Design review of the part built by this model. Coordinates are the model's own, in mm. A direction names the side the tool comes from. Give positions to 0.01 mm unless a question says otherwise; leave off trailing zeros. Loops run counter-clockwise (first coordinate to the right, second up) from the corner with the lowest first, then second, coordinate; pieces in that order, holes last. Notation, with made-up numbers: M 70.25,-33 L 111.25,-33 A19 cw 111.25,-17 Z; hole C 49.5,69.5 d11. An arc over 180 degrees is marked long. Answer as CSV lines item,"result".
```python
from build123d import *

# Parameters (mm, degrees)
SKETCH1_R           = 11
SKETCH1_R_2         = 4
BOSS_EXTRUDE1_DEPTH = 3.5
SKETCH2_R           = 9.4
SKETCH2_R_2         = 5.875
CUT_EXTRUDE1_DEPTH  = 0.5
CUT_EXTRUDE2_START  = -1
SKETCH3_R           = 9.4
SKETCH3_R_2         = 5.875
CUT_EXTRUDE2_DEPTH  = 1
CHAMFER1_SIZE       = 0.5


with BuildPart() as part:
    # Sketch1 → Boss-Extrude1 (new, symmetric)
    with BuildSketch(Plane.XY):
        Circle(SKETCH1_R)
        Circle(SKETCH1_R_2, mode=Mode.SUBTRACT)
    extrude(amount=BOSS_EXTRUDE1_DEPTH, both=True)

    # Sketch2 → Cut-Extrude1 (cut)
    with BuildSketch(Plane.XY.offset(3.5)):
        Circle(SKETCH2_R)
        Circle(SKETCH2_R_2, mode=Mode.SUBTRACT)
    extrude(amount=-CUT_EXTRUDE1_DEPTH, mode=Mode.SUBTRACT)

    # Sketch3 → Cut-Extrude2 (cut)
    with BuildSketch(Plane(origin=(0, 0, -3.5), x_dir=(-1, 0, 0), z_dir=(0, 0, -1)).offset(CUT_EXTRUDE2_START)):
        with Locations(Location((0, 0, 0), (0, 0, 180))):
            Circle(SKETCH3_R)
        with Locations(Location((0, 0, 0), (0, 0, 180))):
            Circle(SKETCH3_R_2, mode=Mode.SUBTRACT)
    extrude(amount=CUT_EXTRUDE2_DEPTH, mode=Mode.SUBTRACT)

    # Chamfer1
    chamfer1_edges = [part.edges().sort_by_distance(p)[0] for p in [
        (-11, 0, -3.5),
        (-11, 0, 3.5),
    ]]
    chamfer(chamfer1_edges, length=CHAMFER1_SIZE)


solid = part.part
```
1. The part is to be moulded in two halves that separate along Y. For faces 4 (the cylindrical face through (-2.38, -10.74, 0.04)), 5 (the flat face through (-2.4, -9.3, -3.5)), 6 (the cylindrical face through (-2.038, -9.176, 3.254)), say which applies: pulls with the +Y half, pulls with the -Y half, needs draft (parallel to the pull), parting line crosses it, or undercut.
Answer block:
face 4,"parting line crosses it"
face 5,"needs draft"
face 6,"undercut"
2. We need section A-A, the plane x = 0. Write out the cut boundary in (y, z) (3 decimals), plus the area to 3 significant figures.
Answer block:
outline,"M -11,-3 L -10.5,-3.5 L -9.4,-3.5 L -9.4,-2.5 L -5.875,-2.5 L -5.875,-3.5 L -4,-3.5 L -4,3.5 L -5.875,3.5 L -5.875,3 L -9.4,3 L -9.4,3.5 L -10.5,3.5 L -11,3 Z; M 4,-3.5 L 5.875,-3.5 L 5.875,-2.5 L 9.4,-2.5 L 9.4,-3.5 L 10.5,-3.5 L 11,-3 L 11,3 L 10.5,3.5 L 9.4,3.5 L 9.4,3 L 5.875,3 L 5.875,3.5 L 4,3.5 Z"
area,"86.9 mm²"
3. For P1, Ø10, axis at x = 1.5, y = 8, coming from the -Z side; P2, Ø1, axis at x = 8.5, z = -0.5, coming from the +Y side; P3, Ø2, axis at y = 7, z = 0, coming from the -X side; P4, Ø3, axis at x = 2.5, z = 0, coming from the +Y side, all flat-tipped, find the tip position at first contact; note any pin that passes through.
Answer block:
P1,"z = -3.5"
P2,"y = 7.55"
P3,"x = -9.22"
P4,"y = 10.95"
4. We need section C-C, the plane z = 1. Write out the cut boundary in (x, y), plus the area to 3 significant figures.
Answer block:
outline,"C 0,0 d22; hole C 0,0 d8"
area,"330 mm²"
5. To check wall thickness, follow L1, parallel to Y at x = 0, z = 0.75; L2, parallel to Y at x = 0, z = -3.2 (3 decimals); L3, parallel to Z at x = 0.25, y = -8.5. State the ranges of each line that lie inside material, in increasing order. Write a range as [from, to].
Answer block:
L1,"[-11, -4], [4, 11]"
L2,"[-10.8, -9.4], [-5.875, -4], [4, 5.875], [9.4, 10.8]"
L3,"[-2.5, 3]"
6. For faces 1 (the flat face through (-2.4, -9.3, 3.5)), 2 (the flat face through (-0.1, -6.1, 3)), 3 (the flat face through (-0.1, 6.1, -2.5)), list the 3-axis set-ups (+Z, -Z, +X, -X, +Y, -Y) from which the entire face can be reached by the end or side of a thin tool; tool diameter is ignored.
Answer block:
face 1,"+Z, +X, -X, +Y, -Y"
face 2,"+Z"
face 3,"-Z"
